Work out the finished part from the listing and answer in its coordinate system (mm). A direction names the side the tool comes from. Coordinates: 2 decimals unless noted, no trailing zeros. Write each loop counter-clockwise with the first axis right and the second up, starting at its lowest first coordinate (ties: lowest second). Pieces come first, ordered by that corner, then holes. Notation, with made-up numbers: (22.5, 29.5) - (49.5, 29.5) arc R26 ccw to (49.5, 63.5) - close; hole circle Ø7 at (17, 87). An arc over 180 degrees is marked (long way). Use a Markdown table: item, result. Add a question column.
(1) A tool of negligible diameter and unlimited length cuts with its end or side. For faces 4 (the face through (2.5, 1.3, 1.9)), 5 (the face through (-2.19, -2.01, 0.03)), 6 (the face through (2, 2, 0)), from which of +Z, -Z, +X, -X, +Y, -Y can it reach the whole face along a straight path? Write none if from no direction.
(2) For a pull along X with two mould halves and no side action, classify faces 1 (the face through (1, 1.4, -6)), 2 (the face through (0.5, 1.7, 2.8)), 3 (the face through (-3.89, 0.69, -5.08)) as released by +X, released by -X, zero draft, split by the parting line, or undercut.
(3) Given pin 1 Ø3 at (x, y) = (2.5, 3) entering from -Z; pin 2 Ø0.6 at (y, z) = (3.5, -4) entering from +X; pin 3 Ø0.6 at (x, z) = (0, 4.5) entering from -Y, each flat-ended and moving along its own axis, determine where each tip first touches the part or whether it passes through.
(4) The part is cut by section B-B, the plane x = 0. Give the vertices of the cut face in (y, z).
(5) Find the intervals of material crossed by line 1 (Z direction, x = 0, y = 2.55); line 2 (X direction, y = 4, z = 2.25), in increasing order. Write a range as from..to.
(6) The part is cut by section A-A, the plane y = 0.25. Give the vertices of the cut face in (x, z).
(7) The part is cut by section C-C, the plane z = 0. Give the vertices of the cut face in (x, y), then the cut area to 3 significant figures.
from build123d import *

# Parameters (mm, degrees)
SKETCH1_R           = 5.75
BOSS_EXTRUDE1_DEPTH = 6
SKETCH2_R           = 6.4
BOSS_EXTRUDE2_DEPTH = 1.4
SKETCH3_R           = 4.9
CUT_EXTRUDE1_DEPTH  = 5
SKETCH4_W           = 0.8
SKETCH4_H           = 6.5
BOSS_EXTRUDE3_DEPTH = 1
BOSS_EXTRUDE4_DEPTH = 1.9
BOSS_EXTRUDE5_START = 4.5
BOSS_EXTRUDE5_DEPTH = 4.5
FILLET1_R           = 0.5


with BuildPart() as part:
    # Sketch1 → Boss-Extrude1 (new body)
    with BuildSketch(Plane(origin=(0, 0, 0), x_dir=(1, 0, 0), z_dir=(0, 1, 0))):
        with Locations(Location((0, 0, 0), (0, 0, 270))):
            Circle(SKETCH1_R)
    extrude(amount=BOSS_EXTRUDE1_DEPTH)

    # Sketch2 → Boss-Extrude2 (add)
    with BuildSketch(Plane(origin=(0, 0, 0), x_dir=(1, 0, 0), z_dir=(0, 1, 0))):
        with Locations(Location((0, 0, 0), (0, 0, 270))):
            Circle(SKETCH2_R)
    extrude(amount=BOSS_EXTRUDE2_DEPTH)

    # Sketch3 → Cut-Extrude1 (cut)
    with BuildSketch(Plane(origin=(0, 0, 0), x_dir=(1, 0, 0), z_dir=(0, 1, 0))):
        with Locations(Location((0, 0, 0), (0, 0, 270))):
            Circle(SKETCH3_R)
    extrude(amount=CUT_EXTRUDE1_DEPTH, mode=Mode.SUBTRACT)

    # Sketch4 → Boss-Extrude3 (add, symmetric)
    with BuildSketch(Plane(origin=(0, 0, 0), x_dir=(0, 0, -1), z_dir=(1, 0, 0))):
        with Locations((2.4, 1.75)):
            Rectangle(SKETCH4_W, SKETCH4_H)
        with Locations((-2.4, 1.75)):
            Rectangle(SKETCH4_W, SKETCH4_H)
    extrude(amount=BOSS_EXTRUDE3_DEPTH, both=True)

    # Sketch5 → Boss-Extrude4 (add, symmetric)
    with BuildSketch(Plane.XY):
        with BuildLine():
            Line((2.9, 5), (2, 5))
            Line((2, 5), (2, -0.9))
            Line((2, -0.9), (1.8, -1.4))
            ThreePointArc((1.8, -1.4), (2.183918232, -2.004066901), (2.7, -2.5))
            Line((2.7, -2.5), (2.9, -2.5))
            Line((2.9, -2.5), (2.9, 5))
        make_face()
        with BuildLine():
            Line((-1.8, -1.4), (-2, -0.9))
            Line((-2, -0.9), (-2, 5))
            Line((-2, 5), (-2.9, 5))
            Line((-2.9, 5), (-2.9, -2.5))
            Line((-2.9, -2.5), (-2.7, -2.5))
            ThreePointArc((-2.7, -2.5), (-2.183918232, -2.004066901), (-1.8, -1.4))
        make_face()
    extrude(amount=BOSS_EXTRUDE4_DEPTH, both=True)

    # Sketch6 → Boss-Extrude5 (add)
    with BuildSketch(Plane.XZ.offset(-5).offset(BOSS_EXTRUDE5_START)):
        with BuildLine():
            Line((-2.9, 0.35), (-4.887484015, 0.35))
            ThreePointArc((-4.887484015, 0.35), (-4.9, 0), (-4.887484015, -0.35))
            Line((-4.887484015, -0.35), (-2.9, -0.35))
            Line((-2.9, -0.35), (-2.9, 0.35))
        make_face()
        with BuildLine():
            Line((0.35, 2.8), (0.35, 4.887484015))
            ThreePointArc((0.35, 4.887484015), (0, 4.9), (-0.35, 4.887484015))
            Line((-0.35, 4.887484015), (-0.35, 2.8))
            Line((-0.35, 2.8), (0.35, 2.8))
        make_face()
        with BuildLine():
            Line((2.9, -0.35), (4.887484015, -0.35))
            ThreePointArc((4.887484015, -0.35), (4.9, 0), (4.887484015, 0.35))
            Line((4.887484015, 0.35), (2.9, 0.35))
            Line((2.9, 0.35), (2.9, -0.35))
        make_face()
        with BuildLine():
            Line((-0.35, -2.8), (-0.35, -4.887484015))
            ThreePointArc((-0.35, -4.887484015), (0, -4.9), (0.35, -4.887484015))
            Line((0.35, -4.887484015), (0.35, -2.8))
            Line((0.35, -2.8), (-0.35, -2.8))
        make_face()
    extrude(amount=-BOSS_EXTRUDE5_DEPTH)

    # Fillet1
    fillet1_edges = [part.edges().sort_by_distance(p)[0] for p in [
        (0, 6, -5.75),
    ]]
    fillet(fillet1_edges, radius=FILLET1_R)


solid = part.part
Model answer:
| question | item | result |
|---|---|---|
| 1 | face 4 | -Y |
| 1 | face 5 | +Z, -Z, -Y |
| 1 | face 6 | none |
| 2 | face 1 | zero draft |
| 2 | face 2 | undercut |
| 2 | face 3 | split by the parting line |
| 3 | pin 1 | z = -5.66 |
| 3 | pin 2 | x = 4.4 |
| 3 | pin 3 | y = 0.5 |
| 4 | outline | (-1.5, -2.8) - (0.5, -2.8) - (0.5, -4.9) - (0, -4.9) - (0, -6.4) - (1.4, -6.4) - (1.4, -5.75) - (5.5, -5.75) arc R0.5 ccw to (6, -5.25) - (6, 5.25) arc R0.5 ccw to (5.5, 5.75) - (1.4, 5.75) - (1.4, 6.4) - (0, 6.4) - (0, 4.9) - (0.5, 4.9) - (0.5, 2.8) - (-1.5, 2.8) - (-1.5, 2) - (5, 2) - (5, -2) - (-1.5, -2) - close |
| 5 | line 1 | -5.75..-2, 2..5.75 |
| 5 | line 2 | -5.29..-4.35, -1..1, 4.35..5.29 |
| 6 | outline | circle Ø12.8 at (0, 0); (-2.9, -1.9) - (-2, -1.9) - (-2, 1.9) - (-2.9, 1.9) - close; (-1, -2.8) - (1, -2.8) - (1, -2) - (-1, -2) - close; (-1, 2) - (1, 2) - (1, 2.8) - (-1, 2.8) - close; (2, -1.9) - (2.9, -1.9) - (2.9, 1.9) - (2, 1.9) - close; hole circle Ø9.8 at (0, 0) |
| 7 | outline | (-6.4, 0) - (-4.9, 0) - (-4.9, 0.5) - (-2.9, 0.5) - (-2.9, -2.5) - (-2.7, -2.5) arc R3 ccw to (-1.8, -1.4) - (-2, -0.9) - (-2, 5) - (2, 5) - (2, -0.9) - (1.8, -1.4) arc R3 ccw to (2.7, -2.5) - (2.9, -2.5) - (2.9, 0.5) - (4.9, 0.5) - (4.9, 0) - (6.4, 0) - (6.4, 1.4) - (5.75, 1.4) - (5.75, 5.5) arc R0.5 ccw to (5.25, 6) - (-5.25, 6) arc R0.5 ccw to (-5.75, 5.5) - (-5.75, 1.4) - (-6.4, 1.4) - close |
| 7 | area | 52.9 mm^2 |
